Geometry check sheet. Reference: the model listing, model coordinates, mm. A direction names the side the tool comes from. Coordinates: 2 decimals unless noted, no trailing zeros. Write each loop counter-clockwise with the first axis right and the second up, starting at its lowest first coordinate (ties: lowest second). Pieces come first, ordered by that corner, then holes. Notation, with made-up numbers: (71, -8.5) -> (86, -8.5) arc R17 cw to (86, 20.5) -> close; hole circle Ø9 at (-13, 69). An arc over 180 degrees is marked (long way). Answer in a Markdown table with one row per item. Add a question column.
1. Depth check by flat-ended pin: P1, Ø10, axis at x = -9, z = -18.5, coming from the +Y side; P2, Ø2, axis at x = -4, y = 2.5, coming from the -Z side; P3, Ø1.4, axis at x = -14, y = 2.5, coming from the -Z side; P4, Ø2, axis at y = 1, z = -18.5, coming from the -X side. Enter the tip coordinate at first touch or a pass-through.
2. Cross-section at D-D on y = 2.5. Record the cut outline in (x, z) (3 decimals).
3. Cross-section at C-C on z = -19.5. Record the cut outline in (x, y), and give its area (3 significant figures).
4. Cross-section at A-A on x = -9. Record the cut outline in (y, z) (3 decimals).
5. Mould release check, pull along Y, two halves, no side actions. Record for faces 3 (the cylindrical face through (-4.06, 2.54, -3.97)), 4 (the flat face through (-9, 0, -12)), 5 (the cylindrical face through (-4.69, 2.21, -0.61)): pulls with the +Y half, pulls with the -Y half, needs draft (parallel to the pull), parting line crosses it, or undercut.
6. Cross-section at B-B on y = 4.2. Record the cut outline in (x, z) (3 decimals), and give its area (3 significant figures).
7. Set-up check for faces 1 (the cylindrical face through (-13.285, 2.725, -0.607)), 2 (the cylindrical face through (-10.93, 2.54, -21.02)): record each of +Z, -Z, +X, -X, +Y, -Y from which the full face is reachable in a straight line by a thin tool's end or side.
8. Scan lines: L1, parallel to X at y = 2.5, z = -0.3; L2, parallel to X at y = 1.7, z = -2.5; L3, parallel to Y at x = -14, z = -0.65. Record each from-to range of solid material in increasing order. Write a range as from..to.
```python
from build123d import *

# Parameters (mm, degrees)
SKETCH1_W                         = 18
SKETCH1_H                         = 24.5
EXTRUDE1_DEPTH                    = 5
SKETCH3_R                         = 1.4732
EXTRUDE2_DEPTH                    = 6
SKETCH4_R                         = 0.75
EXTRUDE3_DEPTH                    = 2.46
FILLET1_R                         = 7.62
F_1_4_20_TAPPED_HOLE1_D           = 5.1054
F_1_4_20_TAPPED_HOLE1_DEPTH       = 16.51
F_1_4_20_TAPPED_HOLE1_CBORE_D     = 6.35
F_1_4_20_TAPPED_HOLE1_CBORE_DEPTH = 12.7
F_1_4_20_TAPPED_HOLE1_TIP         = 1.533816902


with BuildPart() as part:
    # Sketch1 → Extrude1 (new body)
    with BuildSketch(Plane(origin=(0, 0, 0), x_dir=(1, 0, 0), z_dir=(0, 1, 0))):
        with Locations((-9, 12.25)):
            Rectangle(SKETCH1_W, SKETCH1_H)
    extrude(amount=EXTRUDE1_DEPTH)

    # Sketch3 → Extrude2 (cut, through all)
    with BuildSketch(Plane(origin=(0, 5, 0), x_dir=(1, 0, 0), z_dir=(0, 1, 0))):
        with Locations(Location((-14, 2.5, 0), (0, 0, 270))):  # turned: the seam where the file's is
            Circle(SKETCH3_R)
    extrude2 = extrude(amount=-EXTRUDE2_DEPTH, mode=Mode.SUBTRACT)

    # Sketch4 → Extrude3 (cut)
    with BuildSketch(Plane.XY):
        with Locations((-14, 2.5)):
            Circle(SKETCH4_R)
    extrude3 = extrude(amount=-EXTRUDE3_DEPTH, mode=Mode.SUBTRACT)

    # Mirror1: Extrude2, Extrude3 across plane
    add(extrude2.mirror(Plane(origin=(-9, 0, 0), x_dir=(0, 0, 1), z_dir=(1, 0, 0))), mode=Mode.SUBTRACT)
    add(extrude3.mirror(Plane(origin=(-9, 0, 0), x_dir=(0, 0, 1), z_dir=(1, 0, 0))), mode=Mode.SUBTRACT)

    # Fillet1
    fillet1_edges = [part.edges().sort_by_distance(p)[0] for p in [
        (-18, 2.5, -24.5),
        (0, 2.5, -24.5),
    ]]
    fillet(fillet1_edges, radius=FILLET1_R)

    # 1/4-20 Tapped Hole1
    with Locations(Plane(origin=(-9, 5, -18.5), x_dir=(0, 0, 1), z_dir=(0, 1, 0))):
        with Locations((0, 0)):
            CounterBoreHole(F_1_4_20_TAPPED_HOLE1_D / 2, F_1_4_20_TAPPED_HOLE1_CBORE_D / 2, F_1_4_20_TAPPED_HOLE1_CBORE_DEPTH, depth=F_1_4_20_TAPPED_HOLE1_DEPTH)
            with Locations((0, 0, -(F_1_4_20_TAPPED_HOLE1_DEPTH + F_1_4_20_TAPPED_HOLE1_TIP / 2))):  # 118° drill point
                Cone(0, F_1_4_20_TAPPED_HOLE1_D / 2, F_1_4_20_TAPPED_HOLE1_TIP, mode=Mode.SUBTRACT)


solid = part.part
```
Results found:
| question | item | result |
|---|---|---|
| 1 | P1 | stops at y = 5 |
| 1 | P2 | stops at z = -24.04 |
| 1 | P3 | stops at z = -23.92 |
| 1 | P4 | stops at x = -17.97 |
| 2 | outline | (-18, -16.88) arc R7.62 ccw to (-10.38, -24.5) -> (-7.62, -24.5) arc R7.62 ccw to (0, -16.88) -> (0, 0) -> (-3.25, 0) -> (-3.25, -1.232) arc R1.473 cw (long way) to (-4.75, -1.232) -> (-4.75, 0) -> (-13.25, 0) -> (-13.25, -1.232) arc R1.473 cw (long way) to (-14.75, -1.232) -> (-14.75, 0) -> (-18, 0) -> close; hole circle Ø6.35 at (-9, -18.5) |
| 3 | outline | (-17.54, 0) -> (-12.01, 0) -> (-12.01, 5) -> (-17.54, 5) -> close; (-5.99, 0) -> (-0.46, 0) -> (-0.46, 5) -> (-5.99, 5) -> close |
| 3 | area | 55.2 mm^2 |
| 4 | outline | (0, -24.5) -> (5, -24.5) -> (5, -21.675) -> (0, -21.675) -> close; (0, -15.325) -> (5, -15.325) -> (5, 0) -> (0, 0) -> close |
| 5 | face 3 | needs draft |
| 5 | face 4 | pulls with the -Y half |
| 5 | face 5 | undercut |
| 6 | outline | (-18, -16.88) arc R7.62 ccw to (-10.38, -24.5) -> (-7.62, -24.5) arc R7.62 ccw to (0, -16.88) -> (0, 0) -> (-18, 0) -> close; hole circle Ø2.946 at (-14, -2.5); hole circle Ø6.35 at (-9, -18.5); hole circle Ø2.946 at (-4, -2.5) |
| 6 | area | 371 mm^2 |
| 7 | face 1 | +Z |
| 7 | face 2 | +Y, -Y |
| 8 | L1 | x = -18..-14.75, -13.25..-4.75, -3.25..0 |
| 8 | L2 | x = -18..-15.47, -12.53..-5.47, -2.53..0 |
| 8 | L3 | y = 0..1.75, 3.25..5 |
